Source: CAD feature listing. Evaluate the final solid. Frame: model axes, mm. A direction names the side the tool comes from. Round coordinates to 2 decimals unless told otherwise and drop trailing zeros. Order: outer loops, then holes, each group sorted by start corner. A loop starts at its lowest first (then second) coordinate and runs counter-clockwise, first axis right, second up. Notation, with made-up numbers: M 76.25,-12.75 L 128.25,-12.75 A18 cw 128.25,4.25 Z; hole C 74,-8 d9. An arc over 180 degrees is marked long. Answer in a Markdown table with one row per item. Add a question column.
```python
from build123d import *

# Parameters (mm, degrees)
BOSS_EXTRU_1_DEPTH           = 6
ESQUISSE2_R                  = 5.1
ENL_V_MAT_EXTRU_1_DEPTH      = 6
ESQUISSE3_R                  = 3.1
ENL_V_MAT_EXTRU_2_DEPTH      = 76.478473752
ESQUISSE4_R                  = 3.1
ENL_V_MAT_EXTRU_3_DEPTH      = 76.881634801
ENL_V_MAT_EXTRU_4_DEPTH      = 78.42133104
ENL_V_MAT_EXTRU_4_DEPTH_BACK = 78.42133104
ESQUISSE5_W                  = 13.795889793
ESQUISSE5_H                  = 18


with BuildPart() as part:
    # Esquisse1 → Boss.-Extru.1 (new, symmetric)
    with BuildSketch(Plane.XY):
        Polygon((6.25, -15), (8.4, -15), (8.4, 24), (18.25, 24), (18.25, -26), (8.4, -26), (8.4, -75), (6.25, -75), align=None)
    extrude(amount=BOSS_EXTRU_1_DEPTH, both=True)

    # Esquisse2 → Enlèv. mat.-Extru.1 (cut)
    with BuildSketch(Plane(origin=(18.25, 0, 0), x_dir=(0, 0, -1), z_dir=(1, 0, 0))):
        with Locations((0, -20)):
            Circle(ESQUISSE2_R)
    extrude(amount=-ENL_V_MAT_EXTRU_1_DEPTH, mode=Mode.SUBTRACT)

    # Esquisse3 → Enlèv. mat.-Extru.2 (cut, through all)
    with BuildSketch(Plane(origin=(12.25, 0, 0), x_dir=(0, 0, -1), z_dir=(1, 0, 0))):
        with Locations((0, -20)):
            Circle(ESQUISSE3_R)
    extrude(amount=-ENL_V_MAT_EXTRU_2_DEPTH, mode=Mode.SUBTRACT)

    # Esquisse4 → Enlèv. mat.-Extru.3 (cut, through all)
    with BuildSketch(Plane(origin=(8.4, 0, 0), x_dir=(0, 0, -1), z_dir=(1, 0, 0))):
        with Locations(Location((0, -69, 0), (0, 0, 90))):
            Circle(ESQUISSE4_R)
    extrude(amount=-ENL_V_MAT_EXTRU_3_DEPTH, mode=Mode.SUBTRACT)

    # Esquisse5 → Enlèv. mat.-Extru.4 (cut, two sides: drawn at the far end of the back side and taken through both)
    with BuildSketch(Plane.XY.offset(-ENL_V_MAT_EXTRU_4_DEPTH_BACK)):
        with Locations((23.147944897, -1)):
            Rectangle(ESQUISSE5_W, ESQUISSE5_H)
    extrude(amount=ENL_V_MAT_EXTRU_4_DEPTH + ENL_V_MAT_EXTRU_4_DEPTH_BACK, mode=Mode.SUBTRACT)


solid = part.part
```
(1) Cut plane B-B (y = -69). Return loops of the section in (x, z), and give its area (3 significant figures).
(2) Pin query (flat end, axial travel): pin 1 (2 mm diameter, centred on y = -61, z = 0, fed in from +X); pin 2 (3.5 mm diameter, centred on y = 13, z = -3, fed in from -X); pin 3 (0.6 mm diameter, centred on x = 7, z = 1.5, fed in from +Y). Return the tip coordinate at first contact, or that it passes through.
(3) Cut plane A-A (z = 0). Return loops of the section in (x, y).
(4) Access query for faces 5 (the face through (15, -25, 1)), 6 (the face through (17, -10, 0)), 7 (the face through (13, -26, 0)). Directions: +Z, -Z, +X, -X, +Y, -Y. A direction counts if a zero-diameter tool reaches every point of the face in a straight line with its end or side. Return the directions, or none.
(5) Line query: line 1 (Y direction, x = 17.25, z = 0.25); line 2 (Y direction, x = 16, z = 0.25); line 3 (Z direction, x = 6.7, y = -69). Output: solid intervals per line, ascending. Write a range as from..to.
(6) Cut plane C-C (x = 11.25). Return loops of the section in (y, z), and give its area (3 significant figures).
(7) Draft query along Z for faces 1 (the face through (9.292, -23.026, 0.672)), 2 (the face through (8.4, 4, 0)), 3 (the face through (12, -14, -6)), 4 (the face through (12, -14, 6)). Return one class per face: +Z half, -Z half, draft (parallel to the pull), parting line (faces both ways), or undercut.
(8) Cut plane D-D (y = -20). Return loops of the section in (x, z).
Answer list:
| question | item | result |
|---|---|---|
| 1 | outline | M 6.25,-6 L 8.4,-6 L 8.4,-3.1 L 6.25,-3.1 Z; M 6.25,3.1 L 8.4,3.1 L 8.4,6 L 6.25,6 Z |
| 1 | area | 12.5 mm² |
| 2 | pin 1 | x = 8.4 |
| 2 | pin 2 | x = 8.4 |
| 2 | pin 3 | y = -15 |
| 3 | outline | M 6.25,-75 L 8.4,-75 L 8.4,-72.1 L 6.25,-72.1 Z; M 6.25,-65.9 L 8.4,-65.9 L 8.4,-26 L 18.25,-26 L 18.25,-25.1 L 12.25,-25.1 L 12.25,-23.1 L 6.25,-23.1 Z; M 6.25,-16.9 L 12.25,-16.9 L 12.25,-14.9 L 18.25,-14.9 L 18.25,-10 L 16.25,-10 L 16.25,8 L 18.25,8 L 18.25,24 L 8.4,24 L 8.4,-15 L 6.25,-15 Z |
| 4 | face 5 | +X |
| 4 | face 6 | +Z, -Z, +X |
| 4 | face 7 | +Z, -Z, +X, -Y |
| 5 | line 1 | -26..-25.09, -14.91..-10, 8..24 |
| 5 | line 2 | -26..-25.09, -14.91..24 |
| 5 | line 3 | -6..-3.1, 3.1..6 |
| 6 | outline | M -26,-6 L 24,-6 L 24,6 L -26,6 Z; hole C -20,0 d6.2 |
| 6 | area | 570 mm² |
| 7 | face 1 | undercut |
| 7 | face 2 | draft |
| 7 | face 3 | -Z half |
| 7 | face 4 | +Z half |
| 8 | outline | M 6.25,-6 L 18.25,-6 L 18.25,-5.1 L 12.25,-5.1 L 12.25,-3.1 L 6.25,-3.1 Z; M 6.25,3.1 L 12.25,3.1 L 12.25,5.1 L 18.25,5.1 L 18.25,6 L 6.25,6 Z |
